from build123d import *

# Parameters (mm, degrees)
SKETCH_3_W               = 100
SKETCH_3_H               = 3
EXTRUDE_2_DEPTH          = 200
SKETCH_4_R               = 125
CUT_EXTRUDE_3_DEPTH      = 5
SKETCH_5_W               = 62.737548566
SKETCH_5_H               = 5
CUT_EXTRUDE_4_DEPTH      = 207.177108332
PATTERN_CIRCULAR_1_COUNT = 9


with BuildPart() as part:
    # 草圖3 → 填料-伸長2 (new body)
    with BuildSketch(Plane(origin=(0, 0, 0), x_dir=(1, 0, 0), z_dir=(0, 1, 0))):
        with Locations((0, 122.5)):
            Rectangle(SKETCH_3_W, SKETCH_3_H)
    extrude_2 = extrude(amount=-EXTRUDE_2_DEPTH)

    # 草圖4 → 除料-伸長3 (cut)
    with BuildSketch(Plane(origin=(0, -180, 0), x_dir=(-1, 0, 0), z_dir=(0, -1, 0))):
        Circle(SKETCH_4_R)
    extrude(amount=-CUT_EXTRUDE_3_DEPTH, mode=Mode.SUBTRACT)

    # 草圖5 → 除料-伸長4 (cut, through all)
    with BuildSketch(Plane.XY.offset(-121)):
        with Locations((0, -177.5)):
            Rectangle(SKETCH_5_W, SKETCH_5_H)
    cut_extrude_4 = extrude(amount=-CUT_EXTRUDE_4_DEPTH, mode=Mode.SUBTRACT)

    # 環狀複製排列1: 填料-伸長2, 除料-伸長4 ×9 about axis
    pattern_circular_1_axis = Axis((0, 0, 0), (0, 1, 0))
    add([extrude_2.rotate(pattern_circular_1_axis, i * 360 / PATTERN_CIRCULAR_1_COUNT) for i in range(1, PATTERN_CIRCULAR_1_COUNT)])
    add([cut_extrude_4.rotate(pattern_circular_1_axis, i * 360 / PATTERN_CIRCULAR_1_COUNT) for i in range(1, PATTERN_CIRCULAR_1_COUNT)], mode=Mode.SUBTRACT)


solid = part.part
Source: CAD feature listing. Evaluate the final solid. Frame: model axes, mm. A direction names the side the tool comes from. Coordinates: 2 decimals unless noted, no trailing zeros. Loops run counter-clockwise (first coordinate to the right, second up) from the corner with the lowest first, then second, coordinate; pieces in that order, holes last. Notation, with made-up numbers: (86.5, 46) -> (129.5, 46) arc R27 ccw to (129.5, 70) -> close; hole circle Ø11 at (35, 57). An arc over 180 degrees is marked (long way). Answer in a Markdown table with one row per item. Add a question column.
Q1. Contact query for flat-ended pins moving along their axis: pin 1 Ø4 at (y, z) = (-45, -38) entering from +X; pin 2 Ø8 at (x, y) = (-78, -150) entering from +Z; pin 3 Ø2.5 at (y, z) = (-55.5, -122) entering from -X. Output: stop coordinate, or through.
Q2. Reachability of faces 3 (the face through (119.055, -98.6, -21.619)), 4 (the face through (-79, 0, -94)), 5 (the face through (121, -180, -22)) from +Z, -Z, +X, -X, +Y, -Y: full face, straight path, thin tool, end or side. Return the list, or none.
Q3. Section B-B on z = 0.5. Return the cut outline in (x, y).
Q4. Ray query, line 1 along Z through (x, y) = (-88, -110.5); line 2 along Z through (x, y) = (-20, -160); line 3 along X through (y, z) = (-141.5, 9). Return the intervals inside material, ascending.
Q5. Section A-A on z = 73. Return the cut outline in (x, y).
Q6. Pull-direction query (Z, two-part tool) for faces 1 (the face through (78, -180, -94)), 2 (the face through (41.964, -98.6, 113.492)); classes: pulls with the +Z half, pulls with the -Z half, needs draft (parallel to the pull), parting line crosses it, or undercut.
Computed values:
| question | item | result |
|---|---|---|
| 1 | pin 1 | stops at x = 119.57 |
| 1 | pin 2 | stops at z = 105.08 |
| 1 | pin 3 | stops at x = -50 |
| 2 | face 3 | +Y, -Y |
| 2 | face 4 | +Z, -Z, +X, -X, +Y |
| 2 | face 5 | +X, -X |
| 3 | outline | (-126, -200) -> (-122.95, -200) -> (-122.95, -180) -> (-126, -180) -> close; (-126, -175) -> (-122.95, -175) -> (-122.95, 0) -> (-126, 0) -> close; (122.95, -200) -> (126, -200) -> (126, -180) -> (122.95, -180) -> close; (122.95, -175) -> (126, -175) -> (126, 0) -> (122.95, 0) -> close |
| 4 | line 1 | z = -88.03 to -84.11, 89.58 to 95.58, 96.74 to 99.93 |
| 4 | line 2 | z = -124 to -121, 121.49 to 124.68 |
| 4 | line 3 | x = -127.5 to -124.45, 124.45 to 127.5 |
| 5 | outline | (-101.04, -200) -> (-97.57, -200) -> (-97.57, -180) -> (-101.04, -180) -> close; (-101.04, -175) -> (-97.57, -175) -> (-97.57, 0) -> (-101.04, 0) -> close; (97.57, -200) -> (101.04, -200) -> (101.04, -180) -> (97.57, -180) -> close; (97.57, -175) -> (101.04, -175) -> (101.04, 0) -> (97.57, 0) -> close |
| 6 | face 1 | needs draft |
| 6 | face 2 | undercut |
